Verification items for the finished model (mm, model axes). A direction names the side the tool comes from. Coordinates: 2 decimals unless noted, no trailing zeros. Loops run counter-clockwise (first coordinate to the right, second up) from the corner with the lowest first, then second, coordinate; pieces in that order, holes last.
Q1. Access from +Z, -Z, +X, -X, +Y, -Y to the whole of each face (thin tool, end or side, straight path). Record for faces 1 (the face through (0, 0, 0)), 2 (the face through (0, -10, 0)).
Q2. Go/stop test with flat-tipped pins: P1, Ø5, axis at x = -2, y = -2.5, coming from the -Z side; P2, Ø6, axis at x = 7, y = -1.5, coming from the -Z side; P3, Ø6, axis at x = 2, y = -4.5, coming from the -Z side. Record where each tip stops, or that it passes through.
Q3. Material ranges on probe 1 along Y at (x, z) = (11.5, 9.5); probe 2 along Z at (x, y) = (-12.5, 2.5); probe 3 along Z at (x, y) = (11.5, 0.25), recorded low to high.
Q4. Sectioned sample at A-A (x = 0). Enter the section's corners in (y, z), then the cut area to 3 significant figures.
Q5. Sectioned sample at B-B (y = -7). Enter the section's corners in (x, z).
Q6. Mould release check, pull along X, two halves, no side actions. Record for faces 3 (the face through (7.184, 0.789, 13.812)), 4 (the face through (17.327, 3.818, 5.457)), 5 (the face through (-5, 5, -16)): +X half, -X half, draft (parallel to the pull), parting line (faces both ways), or undercut.
Q7. Sectioned sample at C-C (y = -2.5). Enter the section's corners in (x, z).
```python
from build123d import *

# Parameters (mm, degrees)
F0_R     = 18.5
F0_R_2   = 15.5
F1_DEPTH = 5
F1_TAPER = 5
F0_R_3   = 23
F2_DEPTH = 10
F2_TAPER = 15
F3_R     = 5
F4_R     = 0.5


with BuildPart() as f1:
    # F0 (on Front) → F1 (new body)
    with BuildSketch(Plane.XZ):
        Circle(F0_R)
        Circle(F0_R_2, mode=Mode.SUBTRACT)
    extrude(amount=-F1_DEPTH, taper=F1_TAPER)

    # F0 (on Front) → F2 (join)
    with BuildSketch(Plane.XZ):
        Circle(F0_R_3)
        Circle(F0_R, mode=Mode.SUBTRACT)
        Circle(F0_R)
        Circle(F0_R_2, mode=Mode.SUBTRACT)
        Circle(F0_R_2)
    extrude(amount=F2_DEPTH, taper=F2_TAPER)

    # F3
    f3_edges = [f1.edges().sort_by_distance(p)[0] for p in [
        (-20.320508, -10, 0),
    ]]
    fillet(f3_edges, radius=F3_R)

    # F4
    f4_edges = [f1.edges().sort_by_distance(p)[0] for p in [
        (-18.062557, 5, 0),
        (-15.937443, 5, 0),
    ]]
    fillet(f4_edges, radius=F4_R)


solid = f1.part
```
Geometry check:
1. face 1: +Y
1. face 2: +Z, -Z, +X, -X, -Y
2. P1: stops at z = -22.94
2. P2: stops at z = -22.57
2. P3: stops at z = -22.54
3. probe 1: y = -10 to 0
3. probe 2: z = -13.34 to -9.53, 9.53 to 13.34
3. probe 3: z = -14.46 to -10.42, 10.42 to 14.46
4. outline: (-10, -16.48) arc R5 ccw to (-6.29, -21.31) - (0, -23) - (0, -18.5) - (4.54, -18.1) arc R0.5 ccw to (5, -17.6) - (5, -16.4) arc R0.5 ccw to (4.54, -15.9) - (0, -15.5) - (0, 15.5) - (4.54, 15.9) arc R0.5 ccw to (5, 16.4) - (5, 17.6) arc R0.5 ccw to (4.54, 18.1) - (0, 18.5) - (0, 23) - (-6.29, 21.31) arc R5 ccw to (-10, 16.48) - close
4. area: 453 mm2
5. outline: circle Ø42.13 at (0, 0)
6. face 3: undercut
6. face 4: parting line
6. face 5: draft
7. outline: circle Ø44.66 at (0, 0)
